Autodesk Inventor part; units mm, degrees
ref_plane "YZ Plane" through (0, 0, 0) normal (1, 0, 0) x (0, 1, 0)
ref_plane "XZ Plane" through (0, 0, 0) normal (0, 1, 0) x (-1, 0, 0)
ref_plane "XY Plane" through (0, 0, 0) normal (0, 0, 1) x (1, 0, 0)
sketch "Sketch1" plane through (0, 0, 0) normal (0, 1, 0) x (-1, 0, 0)
  line L0 (170, 0) -> (0, 0)
  line L1 (0, 0) -> (0, -80)
  line L2 (0, -80) -> (170, -80)
  line L3 (170, -80) -> (170, 0)
  dimension "d1" = 170
  dimension "d2" = 80
extrude "Extrusion1" add sketch "Sketch1" along normal blind 30
fillet "Fillet1" radius 5 12 edges at (-85, 30, 0) (-85, 30, -80) (0, 30, -40) (-170, 30, -40) (-170, 0, -40) (-170, 15, 0) (-85, 0, 0) (-85, 0, -80) (0, 15, -80) (0, 0, -40) (-170, 15, -80) (0, 15, 0)
sketch "Sketch2" plane through (-165, 5, 0) normal (0, 0, 1) x (1, 0, 0)
  line L0 (148.44, 11.0782) -> (140.5, 11.0782)
  line L1 (140, 10.5782) -> (140, 8.3182)
  line L2 (140.5, 7.8182) -> (148.44, 7.8182)
  line L3 (148.94, 8.3182) -> (148.94, 10.5782)
  line L4 (0, 0) -> (0, 20)
  arc A0 (140.5, 11.0782) -> (140, 10.5782) centre (140.5, 10.5782) ccw
  arc A1 (140, 8.3182) -> (140.5, 7.8182) centre (140.5, 8.3182) ccw
  arc A2 (148.94, 10.5782) -> (148.44, 11.0782) centre (148.44, 10.5782) ccw
  arc A3 (148.44, 7.8182) -> (148.94, 8.3182) centre (148.44, 8.3182) ccw
  line L5 (151.9753, 11.0782) -> (157.8753, 11.0782)
  line L6 (158.3753, 10.5782) -> (158.3753, 9.3282)
  line L7 (156.8753, 8.0782) -> (152.7253, 8.0782)
  line L8 (151.4753, 9.3282) -> (151.4753, 10.5782)
  line L9 (151.4753, 8.0782) -> (151.4753, 8.0782)
  line L10 (151.4753, 8.0782) -> (151.4753, 8.0782) construction
  line L11 (157.1253, 8.0782) -> (156.8753, 8.0782)
  arc A4 (151.9753, 11.0782) -> (151.4753, 10.5782) centre (151.9753, 10.5782) ccw
  arc A5 (158.3753, 10.5782) -> (157.8753, 11.0782) centre (157.8753, 10.5782) ccw
  line L12 (151.4753, 9.3282) -> (152.7253, 8.0782)
  line L13 (151.4753, 9.3282) -> (153.243, 9.3282) construction
  line L14 (158.3753, 9.3282) -> (157.1253, 8.0782)
  point P0 (165, -5)
  point P1 (140, 7.8182)
  point P2 (140, 11.0782)
  point P3 (148.94, 7.8182)
  point P4 (158.3753, 11.0782)
  dimension "d6" = 8.94
  dimension "d7" = 3.26
  dimension "d8" = 140
  dimension "d9" = 0.5
  dimension "d12" = 45
  dimension "d13" = 0
  dimension "d14" = 1.25
  dimension "d15" = 0.5
  dimension "d16" = 6.9
  dimension "d17" = 45
  dimension "d18" = 3
extrude "Extrusion2" cut sketch "Sketch2" against normal blind 5
sketch "Sketch3" plane through (0, 5, -75) normal (1, 0, 0) x (0, 0, -1)
  line L0 (-61.8816, 12.5) -> (-49.8816, 12.5)
  line L1 (-49.3816, 12) -> (-49.3816, 8)
  line L2 (-49.8816, 7.5) -> (-61.8816, 7.5)
  line L3 (-62.3816, 8) -> (-62.3816, 12)
  line L4 (-41.3816, 12.5) -> (-29.3816, 12.5)
  line L5 (-28.8816, 12) -> (-28.8816, 8)
  line L6 (-29.3816, 7.5) -> (-41.3816, 7.5)
  line L7 (-41.8816, 8) -> (-41.8816, 12)
  line L8 (-20.8816, 12.5) -> (-8.8816, 12.5)
  line L9 (-8.3816, 12) -> (-8.3816, 8)
  line L10 (-8.8816, 7.5) -> (-20.8816, 7.5)
  line L11 (-21.3816, 8) -> (-21.3816, 12)
  line L12 (-75, 20) -> (-75, 0)
  line L13 (5, 0) -> (5, 20)
  line L14 (0, 25) -> (-70, 25)
  arc A0 (-61.8816, 12.5) -> (-62.3816, 12) centre (-61.8816, 12) ccw
  arc A1 (-49.3816, 12) -> (-49.8816, 12.5) centre (-49.8816, 12) ccw
  arc A2 (-62.3816, 8) -> (-61.8816, 7.5) centre (-61.8816, 8) ccw
  arc A3 (-49.8816, 7.5) -> (-49.3816, 8) centre (-49.8816, 8) ccw
  arc A4 (-41.3816, 12.5) -> (-41.8816, 12) centre (-41.3816, 12) ccw
  arc A5 (-28.8816, 12) -> (-29.3816, 12.5) centre (-29.3816, 12) ccw
  arc A6 (-41.8816, 8) -> (-41.3816, 7.5) centre (-41.3816, 8) ccw
  arc A7 (-29.3816, 7.5) -> (-28.8816, 8) centre (-29.3816, 8) ccw
  arc A8 (-20.8816, 12.5) -> (-21.3816, 12) centre (-20.8816, 12) ccw
  arc A9 (-8.3816, 12) -> (-8.8816, 12.5) centre (-8.8816, 12) ccw
  arc A10 (-21.3816, 8) -> (-20.8816, 7.5) centre (-20.8816, 8) ccw
  arc A11 (-8.8816, 7.5) -> (-8.3816, 8) centre (-8.8816, 8) ccw
  point P0 (-75, -5)
  point P1 (-49.3816, 7.5)
  point P2 (-49.3816, 12.5)
  point P3 (-62.3816, 7.5)
  point P4 (-28.8816, 7.5)
  point P5 (-28.8816, 12.5)
  point P6 (-41.8816, 7.5)
  point P7 (-8.3816, 7.5)
  point P8 (-8.3816, 12.5)
  point P9 (-21.3816, 7.5)
  point P10 (-49.3816, 10)
  point P11 (-21.3816, 10)
  point P12 (-28.8816, 10)
  point P13 (5, 10)
  point P14 (-62.3816, 10)
  dimension "d21" = 13
  dimension "d22" = 5
  dimension "d23" = 13
  dimension "d24" = 5
  dimension "d25" = 13
  dimension "d26" = 5
  dimension "d27" = 7.5
  dimension "d28" = 7.5
  dimension "d32" = 15
  dimension "d33" = 0.5
extrude "Extrusion3" cut sketch "Sketch3" against normal blind 5
sketch "Sketch4" plane through (-5, 5, -80) normal (0, 0, -1) x (-1, 0, 0)
  circle A0 centre (17.5, 10) radius 5
  line L0 (-5, 20) -> (-5, 0)
  line L1 (0, -5) -> (160, -5)
  circle A1 centre (17.5, 10) radius 4.5
  line L2 (17.5, 7.5) -> (17.5, 12.5) construction
  line L3 (19.5, 11.0782) -> (11.56, 11.0782)
  line L4 (17.75, 7.5) -> (17.75, 12.5)
  line L5 (17.25, 12.5) -> (17.25, 7.5)
  arc A2 (17.25, 7.5) -> (17.75, 7.5) centre (17.5, 7.5) ccw
  arc A3 (17.75, 12.5) -> (17.25, 12.5) centre (17.5, 12.5) ccw
  line L6 (17.5, 10) -> (22.5, 10) construction
  point P0 (-5, -5)
  dimension "d36" = 10
  dimension "d37" = 22.5
  dimension "d38" = 15
  dimension "d39" = 9
  dimension "d40" = 2.5
  dimension "d41" = 90
  dimension "d42" = 0.5
extrude "Extrusion4" cut sketch "Sketch4" against normal blind 0.5
properties part number "Large Battery" material "PET Plastic"
Input: part model. Units: mm. Frame: model coordinates. A direction names the side the tool comes from. Round coordinates to 2 decimals unless told otherwise and drop trailing zeros. Order: outer loops, then holes, each group sorted by start corner. A loop starts at its lowest first (then second) coordinate and runs counter-clockwise, first axis right, second up. Notation, with made-up numbers: (79, 8.25) - (110, 8.25) arc R14 ccw to (110, 14.25) - close; hole circle Ø3 at (25.25, 38.25). An arc over 180 degrees is marked (long way). Answer in a Markdown table with one row per item.
Item 1: Pin query (flat end, axial travel): pin 1 (2.5 mm diameter, centred on x = -3.5, z = -17.5, fed in from -Y); pin 2 (3 mm diameter, centred on x = -1.5, y = 15.5, fed in from +Z); pin 3 (2.5 mm diameter, centred on x = -2, z = -41, fed in from +Y). Return the tip coordinate at first contact, or that it passes through.
Model answer:
| item | result |
|---|---|
| pin 1 | stops at y = 0.01 |
| pin 2 | stops at z = -0.42 |
| pin 3 | stops at y = 29.68 |
Item 2: Reachability of faces 4 (the flat face through (-20, 19, -79.5)), 5 (the flat face through (-2, 17.5, -40)), 6 (the flat face through (-86, 15, 0)), 7 (the flat face through (-21, 14, -5)) from +Z, -Z, +X, -X, +Y, -Y: full face, straight path, thin tool, end or side. Return the list, or none.
Model answer:
| item | result |
|---|---|
| face 4 | -Z |
| face 5 | +X |
| face 6 | +Z, +X, -X, +Y, -Y |
| face 7 | +Z |
Item 3: Line query: line 1 (X direction, y = 15, z = -79.6); line 2 (X direction, y = 4.5, z = -48.5); line 3 (Z direction, x = -43, y = 25.5). Output: solid intervals per line, ascending.
Model answer:
| item | result |
|---|---|
| line 1 | x = -166.96 to -27.5, -27 to -22.75, -22.25 to -18, -17.5 to -3.04 |
| line 2 | x = -169.97 to -0.03 |
| line 3 | z = -79.97 to -0.03 |
Item 4: Section query A-A (x = -20.5). Return the cut outline in (y, z).
Model answer:
| item | result |
|---|---|
| outline | (0, -75) arc R5 ccw to (5, -80) - (10.42, -80) - (10.42, -79.5) - (10.97, -79.5) - (10.97, -80) - (19.03, -80) - (19.03, -79.5) - (19.58, -79.5) - (19.58, -80) - (25, -80) arc R5 ccw to (30, -75) - (30, -5) arc R5 ccw to (25, 0) - (16.08, 0) - (16.08, -5) - (12.82, -5) - (12.82, 0) - (5, 0) arc R5 ccw to (0, -5) - close |
Item 5: Mould query, pull axis Y, two halves, no side actions, for faces 1 (the cylindrical face through (-19.18, 18.04, -79.75)), 2 (the cylindrical face through (-84, 2, -1)), 3 (the cylindrical face through (-169, 15, -2)). Classes: released by +Y, released by -Y, zero draft, split by the parting line, or undercut.
Model answer:
| item | result |
|---|---|
| face 1 | undercut |
| face 2 | released by -Y |
| face 3 | zero draft |
